For this review, take the finished solid that the model builds, in its own axes (mm). Face numbers are marked on the shaded views. A direction names the side the tool comes from. Round coordinates to 2 decimals unless told otherwise and drop trailing zeros. Write each loop counter-clockwise with the first axis right and the second up, starting at its lowest first coordinate (ties: lowest second). Pieces come first, ordered by that corner, then holes. Notation, with made-up numbers: (14, -34) - (39, -34) arc R19 ccw to (39, -3) - close; hole circle Ø6 at (-12, -35). An arc over 180 degrees is marked (long way). One line per item, written item: value. Start each with the question number.
Q1. Mouldability with a two-part tool opening along Y and no side actions: class the marked faces 1, 2 and 3 as +Y half, -Y half, draft (parallel to the pull), parting line (faces both ways), or undercut.
Q2. Tool access review of the marked faces 4 and 5: name each direction out of +Z, -Z, +X, -X, +Y, -Y from which nothing blocks a thin tool from reaching the whole face with its end or side.
Q3. Clearance check with flat-ended pins moving along their axes: pin 1 Ø3 at (x, z) = (4.5, 4.5) entering from -Y; pin 2 Ø0.6 at (y, z) = (-5, 1.5) entering from +X; pin 3 Ø0.8 at (x, y) = (-2.5, -5.5) entering from -Z. State where each tip first meets the part, or that it passes through.
Q4. Add section C-C on x = 7.5. Write out the cut boundary in (y, z).
Q5. For probe 1 along Y at (x, z) = (-2.5, 4.25); probe 2 along Y at (x, z) = (-2.5, 4.35); probe 3 along X at (y, z) = (2.5, 11), list the stretches that pass through material, from the lowest coordinate up.
Q6. Add section D-D on y = -2.25. Write out the cut boundary in (x, z), and give its area (3 significant figures).
Q7. Add section A-A on y = -4.75. Give the number of separate pieces and of enclosed holes in the cut face, and give its area (4 significant figures).
```python
from build123d import *

# Parameters (mm, degrees)
SKETCH_1_W          = 21.4
SKETCH_1_H          = 8.2
EXTRUDE_1_DEPTH     = 12.1
SKETCH_4_R          = 1.25
CUT_EXTRUDE_3_DEPTH = 8
CUT_EXTRUDE_4_DEPTH = 7.8
SKETCH_7_W          = 1
SKETCH_7_H          = 1
EXTRUDE_2_DEPTH     = 8
CHAMFER_1_SIZE      = 0.15
CHAMFER_2_SIZE      = 0.25
SKETCH_8_W          = 1
SKETCH_8_H          = 1
EXTRUDE_3_DEPTH     = 4
CHAMFER_3_SIZE      = 0.15
CHAMFER_4_SIZE      = 0.25
CHAMFER_6_SIZE      = 0.1
CHAMFER_7_SIZE      = 0.2
CHAMFER_8_SIZE      = 0.1
CHAMFER_9_SIZE      = 0.2


with BuildPart() as part:
    # Эскиз1 → Бобышка-Вытянуть1 (new body)
    with BuildSketch(Plane.XY):
        Rectangle(SKETCH_1_W, SKETCH_1_H)
    extrude(amount=EXTRUDE_1_DEPTH)

    # Эскиз4 → Вырез-Вытянуть3 (cut)
    with BuildSketch(Plane.XY.offset(12.1)):
        with Locations((-7.5, 0)):
            Circle(SKETCH_4_R)
        with Locations((-2.5, 0)):
            Circle(SKETCH_4_R)
        with Locations((2.5, 0)):
            Circle(SKETCH_4_R)
        with Locations((7.5, 0)):
            Circle(SKETCH_4_R)
    extrude(amount=-CUT_EXTRUDE_3_DEPTH, mode=Mode.SUBTRACT)

    # Эскиз5 → Вырез-Вытянуть4 (cut)
    with BuildSketch(Plane.XY.offset(12.1)):
        with BuildLine():
            Line((-10.245621634, 0), (-10.245621634, 3.292901982))
            Line((-10.245621634, 3.292901982), (0.278509544, 3.292901982))
            Line((0.278509544, 3.292901982), (5.278509544, 3.292901982))
            Line((5.278509544, 3.292901982), (10.278509544, 3.292901982))
            Line((10.278509544, 3.292901982), (10.278509544, -2.548957219))
            Line((10.278509544, -2.548957219), (9.30582632, -2.548957219))
            ThreePointArc((9.30582632, -2.548957219), (7.5, -3.818893996), (5.69417368, -2.548957219))
            Line((5.69417368, -2.548957219), (4.30582632, -2.548957219))
            ThreePointArc((4.30582632, -2.548957219), (2.5, -3.818893996), (0.69417368, -2.548957219))
            Line((0.69417368, -2.548957219), (-0.69417368, -2.548957219))
            ThreePointArc((-0.69417368, -2.548957219), (-2.5, -3.818893996), (-4.30582632, -2.548957219))
            Line((-4.30582632, -2.548957219), (-5.69417368, -2.548957219))
            ThreePointArc((-5.69417368, -2.548957219), (-7.5, -3.818893996), (-9.30582632, -2.548957219))
            Line((-9.30582632, -2.548957219), (-10.245621634, -2.548957219))
            Line((-10.245621634, -2.548957219), (-10.245621634, 0))
        make_face()
    extrude(amount=-CUT_EXTRUDE_4_DEPTH, mode=Mode.SUBTRACT)

    # Эскиз7 → Бобышка-Вытянуть2 (add)
    with BuildSketch(Plane.XY.offset(4.1)):
        with Locations((-2.5, 0)):
            Rectangle(SKETCH_7_W, SKETCH_7_H)
        with Locations((-7.5, 0)):
            Rectangle(SKETCH_7_W, SKETCH_7_H)
        with Locations((2.5, 0)):
            Rectangle(SKETCH_7_W, SKETCH_7_H)
        with Locations((7.5, 0)):
            Rectangle(SKETCH_7_W, SKETCH_7_H)
    extrude(amount=EXTRUDE_2_DEPTH)

    # Фаска1
    chamfer_1_edges = [part.edges().sort_by_distance(p)[0] for p in [
        (-7, -0.5, 8.1),
        (-7, 0.5, 8.1),
        (-8, 0.5, 8.1),
        (-8, -0.5, 8.1),
        (-2, -0.5, 8.1),
        (-2, 0.5, 8.1),
        (-3, 0.5, 8.1),
        (-3, -0.5, 8.1),
    ]]
    chamfer(chamfer_1_edges, length=CHAMFER_1_SIZE)

    # Фаска2
    # the kernel refuses this chamfer: 0.25 mm, written as the material it takes off along each edge
    with BuildSketch(Plane(origin=(-3, -0.992920747, 12.1), x_dir=(-0.02749587661058555, 0, -0.9996219169112968), z_dir=(0, 1, 0)), Plane(origin=(-3.492920747, 0.5, 12.1), x_dir=(0, 0.027495876610586414, -0.9996219169112968), z_dir=(1, 0, 0)), Plane(origin=(-2, 0.992920747, 12.1), x_dir=(0.027495876610586414, 0, -0.9996219169112968), z_dir=(0, -1, 0)), Plane(origin=(-1.507079253, -0.5, 12.1), x_dir=(0, -0.027495876610586414, -0.9996219169112968), z_dir=(-1, 0, 0)), Plane(origin=(-7, 0.992920747, 12.1), x_dir=(0.02749587661058555, 0, -0.9996219169112968), z_dir=(0, -1, 0)), Plane(origin=(-6.507079253, -0.5, 12.1), x_dir=(0, -0.027495876610586414, -0.9996219169112968), z_dir=(-1, 0, 0)), Plane(origin=(-8, -0.992920747, 12.1), x_dir=(-0.027495876610589005, 0, -0.9996219169112968), z_dir=(0, 1, 0)), Plane(origin=(-8.492920747, 0.5, 12.1), x_dir=(0, 0.027495876610586414, -0.9996219169112968), z_dir=(1, 0, 0))) as chamfer_2_piece_1:
        Polygon((CHAMFER_2_SIZE * 0.999621916911, -CHAMFER_2_SIZE * 0.0274958766106), (-CHAMFER_2_SIZE * 0.0274958766106, -CHAMFER_2_SIZE * 0.999621916911), (0, 0), align=None)
    extrude(amount=1.985841494, mode=Mode.SUBTRACT)

    # Эскиз8 → Бобышка-Вытянуть3 (add)
    with BuildSketch(Plane(origin=(0, -4.1, 0), x_dir=(-1, 0, 0), z_dir=(0, -1, 0))):
        with Locations((2.5, -1.6)):
            Rectangle(SKETCH_8_W, SKETCH_8_H)
        with Locations((7.5, -1.6)):
            Rectangle(SKETCH_8_W, SKETCH_8_H)
        with Locations((-2.5, -1.6)):
            Rectangle(SKETCH_8_W, SKETCH_8_H)
        with Locations((-7.5, -1.6)):
            Rectangle(SKETCH_8_W, SKETCH_8_H)
    extrude(amount=EXTRUDE_3_DEPTH)

    # Фаска3
    chamfer_3_edges = [part.edges().sort_by_distance(p)[0] for p in [
        (8, -0.5, 8.1),
        (8, 0.5, 8.1),
        (7, 0.5, 8.1),
        (7, -0.5, 8.1),
        (-7, -6.1, 1.1),
        (-7, -6.1, 2.1),
        (-8, -6.1, 2.1),
        (-8, -6.1, 1.1),
        (-2, -6.1, 1.1),
        (-2, -6.1, 2.1),
        (-3, -6.1, 2.1),
        (-3, -6.1, 1.1),
        (8, -6.1, 1.1),
        (8, -6.1, 2.1),
        (7, -6.1, 2.1),
        (7, -6.1, 1.1),
    ]]
    chamfer(chamfer_3_edges, length=CHAMFER_3_SIZE)

    # Фаска4
    # the kernel refuses this chamfer: 0.25 mm, written as the material it takes off along each edge
    with BuildSketch(Plane(origin=(-2, -8.1, 2.592920747), x_dir=(0.02749587661058651, 0.9996219169112968, 0), z_dir=(0, 0, -1)), Plane(origin=(-3, -8.1, 0.607079253), x_dir=(-0.027495876610585647, 0.9996219169112968, 0), z_dir=(0, 0, 1)), Plane(origin=(-3.492920747, -8.1, 2.1), x_dir=(0, 0.9996219169112968, 0.027495876610585647), z_dir=(1, 0, 0)), Plane(origin=(-1.507079253, -8.1, 1.1), x_dir=(0, 0.9996219169112968, -0.02749587661058651), z_dir=(-1, 0, 0)), Plane(origin=(-8, -8.1, 0.607079253), x_dir=(-0.0274958766105891, 0.9996219169112968, 0), z_dir=(0, 0, 1)), Plane(origin=(-8.492920747, -8.1, 2.1), x_dir=(0, 0.9996219169112968, 0.027495876610585647), z_dir=(1, 0, 0)), Plane(origin=(-7, -8.1, 2.592920747), x_dir=(0.027495876610585647, 0.9996219169112968, 0), z_dir=(0, 0, -1)), Plane(origin=(-6.507079253, -8.1, 1.1), x_dir=(0, 0.9996219169112968, -0.02749587661058651), z_dir=(-1, 0, 0)), Plane(origin=(8.492920747, -8.1, 1.1), x_dir=(0, 0.9996219169112968, -0.02749587661058651), z_dir=(-1, 0, 0)), Plane(origin=(7, -8.1, 0.607079253), x_dir=(-0.027495876610585647, 0.9996219169112968, 0), z_dir=(0, 0, 1)), Plane(origin=(6.507079253, -8.1, 2.1), x_dir=(0, 0.9996219169112968, 0.027495876610585647), z_dir=(1, 0, 0)), Plane(origin=(8, -8.1, 2.592920747), x_dir=(0.0274958766105891, 0.9996219169112968, 0), z_dir=(0, 0, -1)), Plane(origin=(8.492920747, -0.5, 12.1), x_dir=(0, -0.027495876610586414, -0.9996219169112968), z_dir=(-1, 0, 0)), Plane(origin=(7, -0.992920747, 12.1), x_dir=(-0.02749587661058555, 0, -0.9996219169112968), z_dir=(0, 1, 0)), Plane(origin=(8, 0.992920747, 12.1), x_dir=(0.027495876610589005, 0, -0.9996219169112968), z_dir=(0, -1, 0)), Plane(origin=(6.507079253, 0.5, 12.1), x_dir=(0, 0.027495876610586414, -0.9996219169112968), z_dir=(1, 0, 0))) as chamfer_4_piece_1:
        Polygon((CHAMFER_4_SIZE * 0.999621916911, -CHAMFER_4_SIZE * 0.0274958766106), (-CHAMFER_4_SIZE * 0.0274958766106, -CHAMFER_4_SIZE * 0.999621916911), (0, 0), align=None)
    extrude(amount=1.985841494, mode=Mode.SUBTRACT)

    # Фаска6
    chamfer_6_edges = [part.edges().sort_by_distance(p)[0] for p in [
        (3, -0.5, 8.1),
        (3, 0.5, 8.1),
        (2, 0.5, 8.1),
        (2, -0.5, 8.1),
    ]]
    chamfer(chamfer_6_edges, length=CHAMFER_6_SIZE)

    # Фаска7
    # the kernel refuses this chamfer: 0.2 mm, written as the material it takes off along each edge
    with BuildSketch(Plane(origin=(3, 0.914336598, 12.1), x_dir=(0.02749587661058742, 0, -0.9996219169112966), z_dir=(0, -1, 0)), Plane(origin=(3.414336598, -0.5, 12.1), x_dir=(0, -0.02749587661058634, -0.9996219169112966), z_dir=(-1, 0, 0)), Plane(origin=(2, -0.914336598, 12.1), x_dir=(-0.02749587661058634, 0, -0.9996219169112966), z_dir=(0, 1, 0)), Plane(origin=(1.585663402, 0.5, 12.1), x_dir=(0, 0.02749587661058634, -0.9996219169112966), z_dir=(1, 0, 0))) as chamfer_7_piece_1:
        Polygon((CHAMFER_7_SIZE * 0.999621916911, -CHAMFER_7_SIZE * 0.0274958766106), (-CHAMFER_7_SIZE * 0.0274958766106, -CHAMFER_7_SIZE * 0.999621916911), (0, 0), align=None)
    extrude(amount=1.828673195, mode=Mode.SUBTRACT)

    # Фаска8
    chamfer_8_edges = [part.edges().sort_by_distance(p)[0] for p in [
        (3, -6.1, 1.1),
        (3, -6.1, 2.1),
        (2, -6.1, 2.1),
        (2, -6.1, 1.1),
    ]]
    chamfer(chamfer_8_edges, length=CHAMFER_8_SIZE)

    # Фаска9
    # the kernel refuses this chamfer: 0.2 mm, written as the material it takes off along each edge
    with BuildSketch(Plane(origin=(3, -8.1, 2.514336598), x_dir=(0.027495876610587302, 0.9996219169112966, 0), z_dir=(0, 0, -1)), Plane(origin=(3.414336598, -8.1, 1.1), x_dir=(0, 0.9996219169112968, -0.027495876610586226), z_dir=(-1, 0, 0)), Plane(origin=(2, -8.1, 0.685663402), x_dir=(-0.027495876610586223, 0.9996219169112966, 0), z_dir=(0, 0, 1)), Plane(origin=(1.585663402, -8.1, 2.1), x_dir=(0, 0.9996219169112966, 0.027495876610587302), z_dir=(1, 0, 0))) as chamfer_9_piece_1:
        Polygon((CHAMFER_9_SIZE * 0.999621916911, -CHAMFER_9_SIZE * 0.0274958766106), (-CHAMFER_9_SIZE * 0.0274958766106, -CHAMFER_9_SIZE * 0.999621916911), (0, 0), align=None)
    extrude(amount=1.828673195, mode=Mode.SUBTRACT)


solid = part.part
```
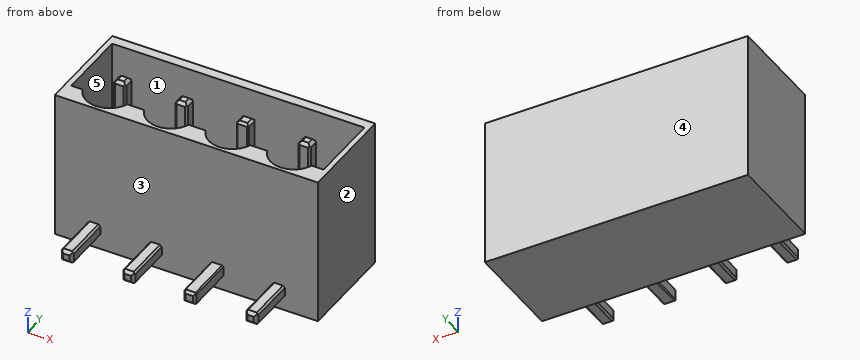
Result set:
1. face 1: undercut
1. face 2: draft
1. face 3: -Y half
2. face 4: +Z, -Z, +X, -X, +Y
2. face 5: +Z
3. pin 1: stops at y = -4.1
3. pin 2: stops at x = 8
3. pin 3: stops at z = 1.1
4. outline: (-8.1, 1.35) - (-7.85, 1.1) - (-4.1, 1.1) - (-4.1, 0) - (4.1, 0) - (4.1, 12.1) - (3.29, 12.1) - (3.29, 4.3) - (1.25, 4.3) - (1.25, 4.1) - (0.5, 4.1) - (0.5, 11.85) - (0.25, 12.1) - (-0.25, 12.1) - (-0.5, 11.85) - (-0.5, 4.1) - (-1.25, 4.1) - (-1.25, 4.3) - (-3.82, 4.3) - (-3.82, 12.1) - (-4.1, 12.1) - (-4.1, 2.1) - (-7.85, 2.1) - (-8.1, 1.85) - close
5. probe 1: y = -4.1 to -1.25, -0.5 to 0.5, 1.25 to 4.1
5. probe 2: y = -4.1 to -3.82, -0.5 to 0.5, 3.29 to 4.1
5. probe 3: x = -10.7 to -10.25, 10.28 to 10.7
6. outline: (-10.7, 0) - (10.7, 0) - (10.7, 12.1) - (10.28, 12.1) - (10.28, 4.3) - (-10.25, 4.3) - (-10.25, 12.1) - (-10.7, 12.1) - close
6. area: 98.9 mm^2
7. separate pieces: 4
7. enclosed holes: 0
7. area: 3.845 mm^2
